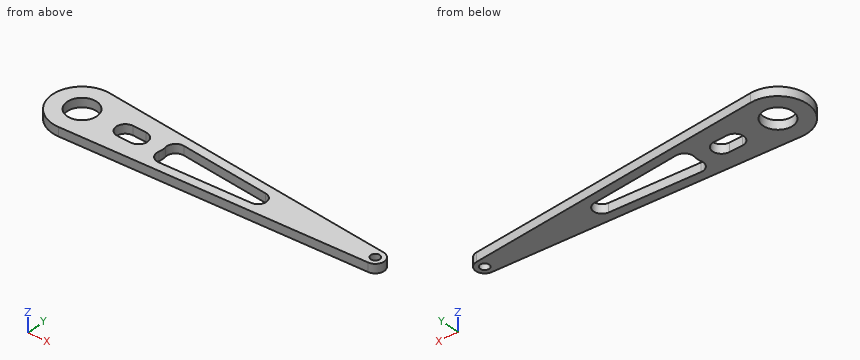
```python
from build123d import *

# Parameters (mm, degrees)
F0_R     = 5
F0_R_2   = 1.5
F1_DEPTH = 1.5


with BuildPart() as f1:
    # F0 (on Top) → F1 (new body, symmetric)
    with BuildSketch(Plane.XY):
        with BuildLine():
            Line((50.21, 2.9926409741), (-49.3, 9.9754699137))
            ThreePointArc((-49.3, 9.9754699137), (-60, 0), (-49.3, -9.9754699137))
            Line((-49.3, -9.9754699137), (50.21, -2.9926409741))
            ThreePointArc((50.21, -2.9926409741), (53, 0), (50.21, 2.9926409741))
        make_face()
        with Locations((-50, 0)):
            Circle(F0_R, mode=Mode.SUBTRACT)
        with BuildLine():
            ThreePointArc((-35.25, -3), (-38.25, 0), (-35.25, 3))
            Line((-35.25, 3), (-30.75, 3))
            ThreePointArc((-30.75, 3), (-27.75, 0), (-30.75, -3))
            Line((-30.75, -3), (-35.25, -3))
        make_face(mode=Mode.SUBTRACT)
        with BuildLine():
            ThreePointArc((-19.5432131994, -4.8799955952), (-22.0323332526, -3.838152351), (-22.6776056819, -1.2180799328))
            ThreePointArc((-22.6776056819, -1.2180799328), (-22.54, 0), (-22.6776056819, 1.2180799328))
            ThreePointArc((-22.6776056819, 1.2180799328), (-22.0323332526, 3.838152351), (-19.5432131994, 4.8799955952))
            Line((-19.5432131994, 4.8799955952), (10.196, 2.7931315758))
            ThreePointArc((10.196, 2.7931315758), (12.8, 0), (10.196, -2.7931315758))
            Line((10.196, -2.7931315758), (-19.5432131994, -4.8799955952))
        make_face(mode=Mode.SUBTRACT)
        with Locations((50, 0)):
            Circle(F0_R_2, mode=Mode.SUBTRACT)
    extrude(amount=F1_DEPTH, both=True)


solid = f1.part
```
Work out the finished part from the listing and answer in its coordinate system (mm). Give positions to 0.01 mm unless a question says otherwise; leave off trailing zeros. Write each loop counter-clockwise with the first axis right and the second up, starting at its lowest first coordinate (ties: lowest second). Pieces come first, ordered by that corner, then holes. Notation, with made-up numbers: (64, 25.5) -> (111, 25.5) arc R16 ccw to (111, 55.5) -> close; hole circle Ø11 at (72.5, -13). An arc over 180 degrees is marked (long way). Write each question's results on one line, items separated by ' | '.
1. Find section C-C on z = -0.95. Determine the outline of the cut face in (x, y), and give its area (3 significant figures).
Data:
outline: (-49.3, -9.98) -> (50.21, -2.99) arc R3 ccw to (50.21, 2.99) -> (-49.3, 9.98) arc R10 ccw (long way) to start; hole circle Ø10 at (-50, 0); hole (-35.25, -3) -> (-30.75, -3) arc R3 ccw to (-30.75, 3) -> (-35.25, 3) arc R3 ccw to start; hole (-22.68, -1.22) arc R3 ccw to (-19.54, -4.88) -> (10.2, -2.79) arc R2.8 ccw to (10.2, 2.79) -> (-19.54, 4.88) arc R3 ccw to (-22.68, 1.22) arc R5.46 cw to start; hole circle Ø3 at (50, 0) | area: 1,070 mm^2
2. Find section B-B on x = -32.5. Determine the outline of the cut face in (y, z).
Data:
outline: (-8.8, -1.5) -> (-3, -1.5) -> (-3, 1.5) -> (-8.8, 1.5) -> close; (3, -1.5) -> (8.8, -1.5) -> (8.8, 1.5) -> (3, 1.5) -> close
3. Find section A-A on y = 0. Determine the outline of the cut face in (x, z), and give its area (3 significant figures).
Data:
outline: (-60, -1.5) -> (-55, -1.5) -> (-55, 1.5) -> (-60, 1.5) -> close; (-45, -1.5) -> (-38.25, -1.5) -> (-38.25, 1.5) -> (-45, 1.5) -> close; (-27.75, -1.5) -> (-22.54, -1.5) -> (-22.54, 1.5) -> (-27.75, 1.5) -> close; (12.8, -1.5) -> (48.5, -1.5) -> (48.5, 1.5) -> (12.8, 1.5) -> close; (51.5, -1.5) -> (53, -1.5) -> (53, 1.5) -> (51.5, 1.5) -> close | area: 162 mm^2
4. Straight lines are drawn through the part: L1, parallel to Y at x = 50, z = -0.7; L2, parallel to Y at x = -50, z = 0.75; L3, parallel to Y at x = 16, z = -0.9. For each, find the intervals that lie inside material, in ascending order.
Data:
L1: -3.01 to -1.5, 1.5 to 3.01 | L2: -10 to -5, 5 to 10 | L3: -5.39 to 5.39
5. Each of these flat-tipped pins is pushed along its axis until it touches: pin 1 Ø1.5 at (y, z) = (-1.5, -0.5) entering from +X; pin 2 Ø0.9 at (x, z) = (-32.5, 0.5) entering from +Y; pin 3 Ø0.9 at (x, z) = (-33.5, 0.5) entering from -Y. Where does it stop, or does it pass through?
Data:
pin 1: x = 52.9 | pin 2: y = 8.83 | pin 3: y = -8.9
6. Find section D-D on y = -6.5. Determine the outline of the cut face in (x, z), and give its area (3 significant figures).
Data:
outline: (-57.6, -1.5) -> (0.23, -1.5) -> (0.23, 1.5) -> (-57.6, 1.5) -> close | area: 173 mm^2
